from build123d import *

# Parameters (mm, degrees)
F1_DEPTH = 45
F2_R     = 6
F3_R     = 8
F4_R     = 5
F5_SIZE  = 15
F6_R     = 5
F7_R     = 5
F8_R     = 8
F9_R     = 6


with BuildPart() as f1:
    # F0 (on Right) → F1 (new body)
    with BuildSketch(Plane.YZ):
        Polygon((13.4, 12.5), (-13.4, 12.5), (-13.4, -12.5), (-11.4, -12.5), (-11.4, 10.5), (11.4, 10.5), (11.4, -12.5), (13.4, -12.5), align=None)
    extrude(amount=F1_DEPTH)

    # F2
    f2_edges = [f1.edges().sort_by_distance(p)[0] for p in [
        (22.5, -11.4, 10.5),
    ]]
    fillet(f2_edges, radius=F2_R)

    # F3
    f3_edges = [f1.edges().sort_by_distance(p)[0] for p in [
        (22.5, -13.4, 12.5),
    ]]
    fillet(f3_edges, radius=F3_R)

    # F4
    f4_edges = [f1.edges().sort_by_distance(p)[0] for p in [
        (0, 12.4, -12.5),
        (45, 12.4, -12.5),
    ]]
    fillet(f4_edges, radius=F4_R)

    # F5
    f5_edges = [f1.edges().sort_by_distance(p)[0] for p in [
        (0, -12.4, -12.5),
    ]]
    chamfer(f5_edges, length=F5_SIZE)

    # F6
    f6_edges = [f1.edges().sort_by_distance(p)[0] for p in [
        (0, -12.4, 2.5),
        (15, -12.4, -12.5),
    ]]
    fillet(f6_edges, radius=F6_R)

    # F7
    f7_edges = [f1.edges().sort_by_distance(p)[0] for p in [
        (45, -12.4, -12.5),
    ]]
    fillet(f7_edges, radius=F7_R)

    # F8
    f8_edges = [f1.edges().sort_by_distance(p)[0] for p in [
        (22.5, 11.4, 10.5),
    ]]
    fillet(f8_edges, radius=F8_R)

    # F9
    f9_edges = [f1.edges().sort_by_distance(p)[0] for p in [
        (22.5, 13.4, 12.5),
    ]]
    fillet(f9_edges, radius=F9_R)


solid = f1.part
The model under review builds one solid part; all positions refer to its coordinate system, in mm. A direction names the side the tool comes from. Give positions to 0.01 mm unless a question says otherwise; leave off trailing zeros. Order: outer loops, then holes, each group sorted by start corner. A loop starts at its lowest first (then second) coordinate and runs counter-clockwise, first axis right, second up. Notation, with made-up numbers: M 37.5,34.5 L 75.5,34.5 A37 cw 75.5,70.5 Z; hole C -9,-11.5 d4. An arc over 180 degrees is marked long. One line per question, with ' | ' between items. Start each with the question number.
1) Consider section A-A, the plane z = -6.5. Give the boundary of the cut face in (x, y).
2) Consider section B-B, the plane x = 28.5. Give the boundary of the cut face in (y, z).
3) Consider section C-C, the plane z = -1.25. Give the boundary of the cut face in (x, y).
4) Mouldability with a two-part tool opening along Y and no side actions: class faces 4 (the face through (15.13, -12.39, -12.11)), 5 (the face through (22.815, -9.689, 8.696)), 6 (the face through (22.815, -11.119, 10.094)), 7 (the face through (22, 11.4, -5)) as pulls with the +Y half, pulls with the -Y half, needs draft (parallel to the pull), parting line crosses it, or undercut.
5) For faces 1 (the face through (7.6, -12.4, -5.1)), 2 (the face through (22, 13.4, -3)), 3 (the face through (22.815, 8.994, 8.219)), list the 3-axis set-ups (+Z, -Z, +X, -X, +Y, -Y) from which the entire face can be reached by the end or side of a thin tool; tool diameter is ignored.
6) Clearance check with flat-ended pins moving along their axes: P1, Ø1.5, axis at x = 21, z = 9, coming from the +Y side; P2, Ø2.5, axis at x = 28, y = -1.5, coming from the -Z side; P3, Ø12, axis at y = 8, z = -2, coming from the -X side. State where each tip first meets the part, or that it passes through.
7) Consider section D-D, the plane y = 1.5. Give the boundary of the cut face in (x, z).
8) Wall thickness on L1, parallel to Y at x = 22, z = -7.75; L2, parallel to Z at x = 24.5, y = -4; L3, parallel to Y at x = 9, z = -9: over which ranges is each line inside the solid? List them lowest first. Write a range as from..to.
Found:
1) outline: M 0,11.4 L 45,11.4 L 45,13.4 L 0,13.4 Z; M 9,-13.4 L 45,-13.4 L 45,-11.4 L 9,-11.4 Z
2) outline: M -13.4,-12.5 L -11.4,-12.5 L -11.4,4.5 A6 cw -5.4,10.5 L 3.4,10.5 A8 cw 11.4,2.5 L 11.4,-12.5 L 13.4,-12.5 L 13.4,6.5 A6 ccw 7.4,12.5 L -5.4,12.5 A8 ccw -13.4,4.5 Z
3) outline: M 0,11.4 L 45,11.4 L 45,13.4 L 0,13.4 Z; M 3.75,-13.4 L 45,-13.4 L 45,-11.4 L 3.75,-11.4 Z
4) face 4: needs draft | face 5: undercut | face 6: pulls with the -Y half | face 7: undercut
5) face 1: -Z, -X, -Y | face 2: +Z, -Z, +X, -X, +Y | face 3: -Z, +X, -X
6) P1: stops at y = 13.14 | P2: stops at z = 10.5 | P3: stops at x = 0
7) outline: M 0,10.5 L 45,10.5 L 45,12.5 L 0,12.5 Z
8) L1: y = -13.4..-11.4, 11.4..13.4 | L2: z = 10.5..12.5 | L3: y = 11.4..13.4
